The listing builds one solid part. Answer for the finished solid, in the listing's coordinates (mm). Face numbers are marked on the shaded views. A direction names the side the tool comes from. Coordinates: 2 decimals unless noted, no trailing zeros. Loops run counter-clockwise (first coordinate to the right, second up) from the corner with the lowest first, then second, coordinate; pieces in that order, holes last. Notation, with made-up numbers: (55, -1) - (83, -1) arc R22 ccw to (83, 14) - close; hole circle Ø9 at (2.5, 81). An arc over 180 degrees is marked (long way). Write each question's results on one line, items separated by ' | '. Start each with the question number.
(1) Find section A-A on z = 0.9. Determine the outline of the cut face in (x, y), then the cut area to 3 significant figures.
(2) Find section B-B on y = 0. Determine the outline of the cut face in (x, z), then the cut area to 3 significant figures.
(3) Given pin 1 Ø0.9 at (x, z) = (2, 2) entering from -Y; pin 2 Ø1.5 at (x, z) = (2, 1) entering from +Y; pin 3 Ø2.5 at (y, z) = (2.5, 1) entering from -X, each flat-ended and moving along its own axis, determine where each tip first touches the part or whether it passes through.
(4) Find section D-D on z = 5.1. Determine the outline of the cut face in (x, y), then the cut area to 3 significant figures.
(5) For the marked faces 1, 2, 3 and 4, determine the directions among +Z, -Z, +X, -X, +Y, -Y from which every point of the face is accessible in a straight line to the end or side of a thin tool.
(6) Consider line 1 (Z direction, x = -1.5, y = -7.5); line 2 (Z direction, x = 2, y = -3.5); line 3 (Y direction, x = -1, z = 1.4). Determine where each line is inside the solid, lowest interval first. Write a range as from..to.
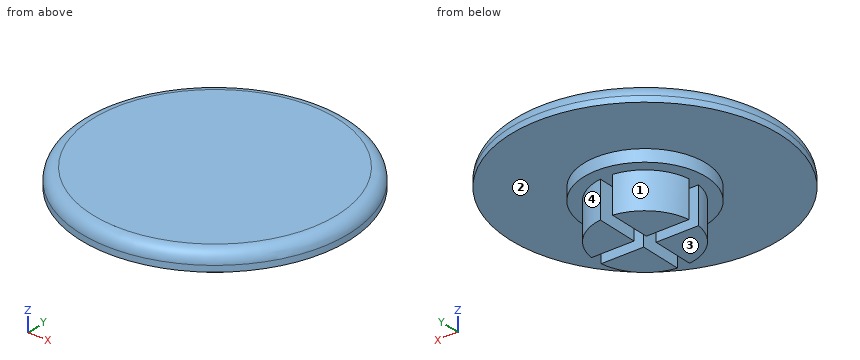
from build123d import *

# Parameters (mm, degrees)
F3_DEPTH = 3
F4_R     = 1


with BuildPart() as f1:
    # F0 (on Front) → F1 (revolve)
    with BuildSketch(Plane.XZ):
        Polygon((0, 5.5), (0, 0), (4, 0), (4, 3), (5, 3), (5, 4), (11, 4), (11, 5.5), align=None)
    revolve(axis=Axis((0, 0, 5.302473), (0, 0, 1)))

    # F2 (on face) → F3 (cut, through all)
    with BuildSketch(Plane(origin=(0, 0, 0), x_dir=(1, 0, 0), z_dir=(0, 0, -1))):
        Polygon((-0.5, -6.403249), (0.5, -6.403249), (0.5, -0.5), (5.621079, -0.5), (5.621079, 0.5), (0.5, 0.5), (0.5, 6.403249), (-0.5, 6.403249), (-0.5, 0.5), (-5.621079, 0.5), (-5.621079, -0.5), (-0.5, -0.5), align=None)
    extrude(amount=-F3_DEPTH, mode=Mode.SUBTRACT)

    # F4
    f4_edges = [f1.edges().sort_by_distance(p)[0] for p in [
        (-11, 0, 5.5),
    ]]
    fillet(f4_edges, radius=F4_R)


solid = f1.part
Values:
1) outline: (-3.97, -0.5) arc R4 ccw to (-0.5, -3.97) - (-0.5, -0.5) - close; (-3.97, 0.5) - (-0.5, 0.5) - (-0.5, 3.97) arc R4 ccw to start; (0.5, -3.97) arc R4 ccw to (3.97, -0.5) - (0.5, -0.5) - close; (0.5, 0.5) - (3.97, 0.5) arc R4 ccw to (0.5, 3.97) - close | area: 35.3 mm²
2) outline: (-11, 4) - (-5, 4) - (-5, 3) - (5, 3) - (5, 4) - (11, 4) - (11, 4.5) arc R1 ccw to (10, 5.5) - (-10, 5.5) arc R1 ccw to (-11, 4.5) - close | area: 42.6 mm²
3) pin 1: stops at y = -3.69 | pin 2: stops at y = 3.8 | pin 3: stops at x = -3.8
4) outline: circle Ø21.6 at (0, 0) | area: 366 mm²
5) face 1: -Z, -X, +Y | face 2: -Z | face 3: -Z, +X, -X, +Y, -Y | face 4: -Z, +X, +Y
6) line 1: z = 4..5.5 | line 2: z = 3..5.5 | line 3: y = -3.87..-0.5, 0.5..3.87
